Geometry: final body of the model. Coordinates: model frame, mm. A direction names the side the tool comes from. Give positions to 0.01 mm unless a question says otherwise; leave off trailing zeros. Write each loop counter-clockwise with the first axis right and the second up, starting at its lowest first coordinate (ties: lowest second). Pieces come first, ordered by that corner, then holes. Notation, with made-up numbers: (56, -30) - (91, -30) arc R7 ccw to (91, -23) - close; hole circle Ø5 at (78.25, -9). An arc over 180 degrees is marked (long way). Use CSV: the item, a comma, the result in double quotes. Start each with the question number.
(1) First-contact query: pin 1 Ø3 at (x, z) = (2, 2) entering from +Y. Flat tip, straight axial feed; report the tip coordinate or a pass-through.
(2) Section B-B on y = -0.65. Output: boundary loops of the cut face in (x, z), and give its area (3 significant figures).
(3) Section C-C on x = 11.5. Output: boundary loops of the cut face in (y, z).
(4) Reachability of faces 4 (the cylindrical face through (0, 1, 1)), 5 (the flat face through (12.9, -0.8, 2)), 6 (the flat face through (11.056, 0, 7)), 7 (the flat face through (12.9, 0.8, 2)) from +Z, -Z, +X, -X, +Y, -Y: full face, straight path, thin tool, end or side. Return the list, or none.
(5) Draft query along X for faces 1 (the flat face through (5, 1, 16)), 2 (the flat face through (-1, 0, 9)), 3 (the flat face through (0.79, 0.84, 2)). Return one class per face: released by +X, released by -X, zero draft, split by the parting line, or undercut.
(6) Line query: probe 1 along X at (y, z) = (0.6, 8.75); probe 2 along Z at (x, y) = (8, 0.45); probe 3 along X at (y, z) = (0.2, 14.75). Output: solid intervals per line, ascending. Write a range as [from, to].
(7) Section A-A on z = 10.5. Output: boundary loops of the cut face in (x, y).
(8) Section D-D on x = 6.25. Output: boundary loops of the cut face in (y, z).
Autodesk Inventor part; units mm, degrees
ref_plane "YZ Plane" through (0, 0, 0) normal (1, 0, 0) x (0, 1, 0)
ref_plane "XZ Plane" through (0, 0, 0) normal (0, 1, 0) x (-1, 0, 0)
ref_plane "XY Plane" through (0, 0, 0) normal (0, 0, 1) x (1, 0, 0)
sketch "Esboço1" plane through (0, 0, 0) normal (0, 0, 1) x (1, 0, 0)
  circle A0 centre (0, 0) radius 1
  line L0 (0, 0) -> (12.0565, 0) construction
  circle A1 centre (12.0565, 0) radius 1
  dimension "d0" = 2
  dimension "d1" = 12.0565
  dimension "d2" = 2
extrude "Extrusão1" add sketch "Esboço1" along normal blind 2
sketch "Esboço2" plane through (0, 0, 2) normal (0, 0, 1) x (1, 0, 0)
  line L0 (-1, 1) -> (1, 1)
  line L1 (1, 1) -> (1, -1)
  line L2 (1, -1) -> (-1, -1)
  line L3 (-1, -1) -> (-1, 1)
  circle A0 centre (0, 0) radius 1
  line L4 (-1, 1) -> (1, -1) construction
  line L5 (1, 1) -> (-1, -1) construction
  circle A1 centre (12.0565, 0) radius 1
  line L6 (0, 0) -> (12.0565, 0) construction
  line L7 (11.0565, 1) -> (13.0565, 1)
  line L8 (13.0565, 1) -> (13.0565, -1)
  line L9 (13.0565, -1) -> (11.0565, -1)
  line L10 (11.0565, -1) -> (11.0565, 1)
  line L11 (11.0565, 1) -> (13.0565, -1) construction
  line L12 (13.0565, 1) -> (11.0565, -1) construction
extrude "Extrusão2" add sketch "Esboço2" along normal blind 15
sketch "Esboço3" plane through (0, 0, 17) normal (0, 0, 1) x (1, 0, 0)
  line L0 (1, 0) -> (1, 1)
  line L1 (12.0565, 1) -> (11.0565, 1)
  line L2 (1, 1) -> (11.0565, 1)
  line L3 (11.0565, 1) -> (11.0565, -1)
  line L4 (11.0565, -1) -> (1, -1)
  line L5 (1, -1) -> (1, 1)
  point P0 (0, 0)
  dimension "d7" = 2
extrude "Extrusão3" add sketch "Esboço3" against normal blind 2
fillet "Arredondamento1" radius 2 2 edges at (11.0565, 0, 15) (1, 0, 15)
properties part number "Trem_Pouso"
Check values:
1,pin 1,"stops at y = 1"
2,outline,"(-1, 2) - (-0.76, 2) - (-0.76, 0) - (0.76, 0) - (0.76, 2) - (1, 2) - (1, 13) arc R2 cw to (3, 15) - (9.06, 15) arc R2 cw to (11.06, 13) - (11.06, 2) - (11.3, 2) - (11.3, 0) - (12.82, 0) - (12.82, 2) - (13.06, 2) - (13.06, 17) - (-1, 17) - close"
2,area,"87.9 mm²"
3,outline,"(-1, 2) - (-0.83, 2) - (-0.83, 0) - (0.83, 0) - (0.83, 2) - (1, 2) - (1, 17) - (-1, 17) - close"
4,face 4,"-Z"
4,face 5,"-Z, +X, -Y"
4,face 6,"-Z, +Y, -Y"
4,face 7,"-Z, +X, +Y"
5,face 1,"zero draft"
5,face 2,"released by -X"
5,face 3,"undercut"
6,probe 1,"x = [-1, 1], [11.06, 13.06]"
6,probe 2,"z = [15, 17]"
6,probe 3,"x = [-1, 2.03], [10.02, 13.06]"
7,outline,"(-1, -1) - (1, -1) - (1, 1) - (-1, 1) - close; (11.06, -1) - (13.06, -1) - (13.06, 1) - (11.06, 1) - close"
8,outline,"(-1, 15) - (1, 15) - (1, 17) - (-1, 17) - close"
